from build123d import *

# Parameters (mm, degrees)
F1_DEPTH  = 2
F2_W      = 2
F2_H      = 134
F3_DEPTH  = 30
F4_R      = 1
F5_W      = 8
F5_H      = 130
F6_DEPTH  = 2
F7_R      = 1
F8_W      = 124
F8_H      = 2
F9_DEPTH  = 9
F10_R     = 1
F11_W     = 0.5
F11_H     = 1
F12_DEPTH = 135.001
F13_R     = 1.5
F13_R_2   = 6.5
F13_W     = 18
F13_H     = 10
F14_DEPTH = 3
F15_R     = 1.1
F15_R_2   = 1.5
F16_DEPTH = 3
F17_R     = 1.1
F18_DEPTH = 134.001
F19_R     = 1.5
F19_W     = 18
F19_H     = 10
F20_DEPTH = 3


with BuildPart() as f1:
    # F0 (on Top) → F1 (new body)
    with BuildSketch(Plane.XY):
        Polygon((62.5, -67), (67.5, -67), (67.5, 67), (62.5, 67), (62.5, 64), (62, 64), (62, 67), (-62, 67), (-62, 64), (-62.5, 64), (-62.5, 67), (-67.5, 67), (-67.5, -67), (-62.5, -67), (-62.5, -64), (-62, -64), (-62, -67), (62, -67), (62, -64), (62.5, -64), align=None)
    extrude(amount=F1_DEPTH)

    # F2 (on face) → F3 (join)
    with BuildSketch(Plane.XY.offset(2)):
        with Locations((66.5, 0)):
            Rectangle(F2_W, F2_H)
        with Locations((-66.5, 0)):
            Rectangle(F2_W, F2_H)
    extrude(amount=F3_DEPTH)

    # F4
    f4_edges = [f1.edges().sort_by_distance(p)[0] for p in [
        (-67.5, 0, 0),
        (67.5, 0, 0),
        (-65.5, 0, 2),
        (65.5, 0, 2),
    ]]
    fillet(f4_edges, radius=F4_R)

    # F5 (on face) → F6 (join)
    with BuildSketch(Plane.XY.offset(32)):
        with Locations((-63.5, 0)):
            Rectangle(F5_W, F5_H)
        with Locations((63.5, 0)):
            Rectangle(F5_W, F5_H)
    extrude(amount=F6_DEPTH)

    # F7
    f7_edges = [f1.edges().sort_by_distance(p)[0] for p in [
        (-67.5, 0, 34),
        (67.5, 0, 34),
        (-65.5, 0, 32),
        (65.5, 0, 32),
    ]]
    fillet(f7_edges, radius=F7_R)

    # F8 (on face) → F9 (join)
    with BuildSketch(Plane.XY.offset(2)):
        with Locations((0, -66)):
            Rectangle(F8_W, F8_H)
        with Locations((0, 66)):
            Rectangle(F8_W, F8_H)
    extrude(amount=F9_DEPTH)

    # F10
    f10_edges = [f1.edges().sort_by_distance(p)[0] for p in [
        (0, -67, 0),
        (0, -65, 2),
        (0, 65, 2),
        (0, 67, 0),
    ]]
    fillet(f10_edges, radius=F10_R)

    # F11 (on face) → F12 (cut, through all)
    with BuildSketch(Plane(origin=(-67.5, 0, 0), x_dir=(0, -1, 0), z_dir=(-1, 0, 0))):
        with Locations((65.25, 31.5)):
            Rectangle(F11_W, F11_H)
        with Locations((-65.25, 31.5)):
            Rectangle(F11_W, F11_H)
    extrude(amount=-F12_DEPTH, mode=Mode.SUBTRACT)

    # F13 (on face) → F14 (cut)
    with BuildSketch(Plane(origin=(-67.5, 0, 0), x_dir=(0, -1, 0), z_dir=(-1, 0, 0))):
        with Locations((-55, 15)):
            Circle(F13_R)
        with Locations((-30, 15)):
            Circle(F13_R)
        with Locations((0, 17)):
            Circle(F13_R_2)
        with Locations((-15, 17)):
            Circle(F13_R)
        with Locations((-42.5, 15)):
            Rectangle(F13_W, F13_H)
    extrude(amount=-F14_DEPTH, mode=Mode.SUBTRACT)

    # F15 (on face) → F16 (cut)
    with BuildSketch(Plane.XY.offset(2)):
        with Locations((-33, 30)):
            Circle(F15_R)
        with Locations((19, 30)):
            Circle(F15_R)
        with Locations((-33, -30)):
            Circle(F15_R)
        with Locations((19, -30)):
            Circle(F15_R)
        with Locations((-45, -16.5)):
            Circle(F15_R)
        with Locations((-61, -47.5)):
            Circle(F15_R)
        with Locations((-59.5, 59)):
            Circle(F15_R_2)
        with Locations((59.5, 59)):
            Circle(F15_R_2)
        with Locations((-59.5, -59)):
            Circle(F15_R_2)
        with Locations((59.5, -59)):
            Circle(F15_R_2)
        with Locations((35.5, 30)):
            Circle(F15_R)
        with Locations((51.5, 30)):
            Circle(F15_R)
        with Locations((35.5, -53)):
            Circle(F15_R)
        with Locations((51.5, -53)):
            Circle(F15_R)
    extrude(amount=-F16_DEPTH, mode=Mode.SUBTRACT)

    # F17 (on face) → F18 (cut, through all)
    with BuildSketch(Plane.XZ.offset(67)):
        with Locations((54, 7)):
            Circle(F17_R)
        with Locations((-54, 7)):
            Circle(F17_R)
    extrude(amount=-F18_DEPTH, mode=Mode.SUBTRACT)

    # F19 (on face) → F20 (cut)
    with BuildSketch(Plane.YZ.offset(67.5)):
        with Locations((30, 15)):
            Circle(F19_R)
        with Locations((55, 15)):
            Circle(F19_R)
        with Locations((42.5, 15)):
            Rectangle(F19_W, F19_H)
    extrude(amount=-F20_DEPTH, mode=Mode.SUBTRACT)


solid = f1.part
For this review, take the finished solid that the model builds, in its own axes (mm). A direction names the side the tool comes from. Round coordinates to 2 decimals unless told otherwise and drop trailing zeros. Loops run counter-clockwise (first coordinate to the right, second up) from the corner with the lowest first, then second, coordinate; pieces in that order, holes last. Notation, with made-up numbers: (-14, 17.25) - (28, 17.25) arc R20 cw to (28, 32.25) - close; hole circle Ø11 at (-36, 86). An arc over 180 degrees is marked (long way). One line per item, written item: value. Start each with the question number.
Item 1: Take a section at C-C (x = 15). Give the boundary of the cut face in (y, z).
Item 2: Take a section at A-A (y = 0). Give the boundary of the cut face in (x, z), plus the area to 3 significant figures.
Item 3: Take a section at B-B (z = 29). Give the boundary of the cut face in (x, y), plus the area to 3 significant figures.
Item 4: For L1, parallel to Y at x = 19, z = 1.15; L2, parallel to X at y = 53.5, z = 12; L3, parallel to Z at x = 54, y = 65.8, list the stretches that pass through material, from the lowest coordinate up.
Item 5: For faces 1 (the cylindrical face through (61, 59, 1)), 2 (the cylindrical face through (-66.51, 53.57, 15.45)), list the 3-axis set-ups (+Z, -Z, +X, -X, +Y, -Y) from which the entire face can be reached by the end or side of a thin tool; tool diameter is ignored.
Item 6: Clearance check with flat-ended pins moving along their axes: pin 1 Ø6 at (x, y) = (54, -50) entering from +Z; pin 2 Ø1 at (x, y) = (-14, 66.5) entering from +Z; pin 3 Ø10 at (x, z) = (-49.5, 20.5) entering from +Y; pin 4 Ø3.5 at (x, z) = (61.5, 32) entering from -Y. State where each tip first meets the part, or that it passes through.
Item 7: The part is to be moulded in two halves that separate along Y. For faces 3 (the flat face through (67.5, -1, 17)), 4 (the flat face through (-66, -67, 16)), 5 (the cylindrical face through (-66.51, 16.11, 18.01)), say which applies: +Y half, -Y half, draft (parallel to the pull), parting line (faces both ways), or undercut.
Answer below:
1. outline: (-67, 1) arc R1 ccw to (-66, 0) - (66, 0) arc R1 ccw to (67, 1) - (67, 11) - (65, 11) - (65, 3) arc R1 cw to (64, 2) - (-64, 2) arc R1 cw to (-65, 3) - (-65, 11) - (-67, 11) - close
2. outline: (-67.5, 1) arc R1 ccw to (-66.5, 0) - (66.5, 0) arc R1 ccw to (67.5, 1) - (67.5, 33) arc R1 ccw to (66.5, 34) - (59.5, 34) - (59.5, 32) - (64.5, 32) arc R1 cw to (65.5, 31) - (65.5, 3) arc R1 cw to (64.5, 2) - (-64.5, 2) arc R1 cw to (-65.5, 3) - (-65.5, 10.5) - (-67.5, 10.5) - close; (-67.5, 23.5) - (-65.5, 23.5) - (-65.5, 31) arc R1 cw to (-64.5, 32) - (-59.5, 32) - (-59.5, 34) - (-66.5, 34) arc R1 ccw to (-67.5, 33) - close
2. area: 396 mm2
3. outline: (-67.5, -67) - (-65.5, -67) - (-65.5, 67) - (-67.5, 67) - close; (65.5, -67) - (67.5, -67) - (67.5, 67) - (65.5, 67) - close
3. area: 536 mm2
4. L1: y = -67 to -31.1, -28.9 to 28.9, 31.1 to 67
4. L2: x = -67.5 to -65.5, 65.5 to 67.5
4. L3: z = 0 to 5.9, 8.1 to 11
5. face 1: -Z
5. face 2: +X, -X
6. pin 1: stops at z = 2
6. pin 2: stops at z = 11
6. pin 3: passes through
6. pin 4: stops at y = -65
7. face 3: draft
7. face 4: -Y half
7. face 5: undercut
